Here's how the part is built. I have some questions about the finished solid (model axes, mm). A direction names the side the tool comes from. Round coordinates to 2 decimals unless told otherwise and drop trailing zeros. Loops run counter-clockwise (first coordinate to the right, second up) from the corner with the lowest first, then second, coordinate; pieces in that order, holes last. Notation, with made-up numbers: M 82.5,33 L 133.5,33 A33 cw 133.5,70 Z; hole C 8.25,14 d7. An arc over 180 degrees is marked long. Use a Markdown table: item, result.
```python
from build123d import *

# Parameters (mm, degrees)
F0_W            = 30
F0_H            = 40
F1_DEPTH        = 2
F2_W            = 14
F2_H            = 8
F3_DEPTH        = 10
F5_DEPTH        = 10
F6_R            = 5
F7_R            = 2.5
F8_W            = 15
F8_H            = 40
F8_W_2          = 9
F8_H_2          = 34
F9_DEPTH        = 2
F10_W           = 0.8
F10_H           = 34
F11_DEPTH       = 10
F12_W           = 9
F12_H           = 8
F13_DEPTH       = 2
F14_W           = 5
F14_H           = 2.75
F14_H_2         = 4
F15_DEPTH       = 10
F17_DEPTH       = 1
F18_W           = 9
F18_H           = 6
F19_DEPTH       = 2
F20_R           = 1
F22_D           = 5.5
F22_CBORE_D     = 6.5
F22_CBORE_DEPTH = 0


with BuildPart() as f1:
    # F0 (on Top) → F1 (new body)
    with BuildSketch(Plane.XY):
        Rectangle(F0_W, F0_H)
    extrude(amount=F1_DEPTH)

    # F2 (on face) → F3 (cut)
    with BuildSketch(Plane.XY.offset(2)):
        with Locations((0, 8)):
            Rectangle(F2_W, F2_H)
    extrude(amount=-F3_DEPTH, mode=Mode.SUBTRACT)

    # F4 (on face) → F5 (cut)
    with BuildSketch(Plane.XY.offset(2)):
        Polygon((-1, -4), (-7, -4), (-7, -20), (7, -20), align=None)
        Polygon((15, -4), (7, -4), (15, -20), align=None)
    extrude(amount=-F5_DEPTH, mode=Mode.SUBTRACT)

    # F6
    f6_edges = [f1.edges().sort_by_distance(p)[0] for p in [
        (15, -4, 1),
        (15, 20, 1),
        (-1, -4, 1),
    ]]
    fillet(f6_edges, radius=F6_R)

    # F7
    f7_edges = [f1.edges().sort_by_distance(p)[0] for p in [
        (7, 12, 1),
        (7, 4, 1),
    ]]
    fillet(f7_edges, radius=F7_R)

    # F8 (on face) → F9 (join)
    with BuildSketch(Plane.XY.offset(2)):
        with Locations((-22.5, 0)):
            Rectangle(F8_W, F8_H)
        with Locations((-22.5, 0)):
            Rectangle(F8_W_2, F8_H_2, mode=Mode.SUBTRACT)
    extrude(amount=-F9_DEPTH)

    # F10 (on face) → F11 (cut)
    with BuildSketch(Plane.XY.offset(2)):
        with Locations((-14.8, 0)):
            Rectangle(F10_W, F10_H)
    extrude(amount=-F11_DEPTH, mode=Mode.SUBTRACT)

    # F12 (on face) → F13 (join)
    with BuildSketch(Plane.XY.offset(2)):
        with Locations((-22.5, -12.75)):
            Rectangle(F12_W, F12_H)
        with Locations((-22.5, -4.25)):
            Rectangle(F12_W, F12_H)
        with Locations((-22.5, 4.25)):
            Rectangle(F12_W, F12_H)
        with Locations((-22.5, 12.75)):
            Rectangle(F12_W, F12_H)
    extrude(amount=-F13_DEPTH)

    # F14 (on face) → F15 (cut)
    with BuildSketch(Plane.XY.offset(2)):
        with Locations((-22.5, -15.375)):
            Rectangle(F14_W, F14_H)
        with Locations((-22.5, -10.125)):
            Rectangle(F14_W, F14_H)
        Polygon((-27, -2.25), (-27, -6.25), (-21, -2.25), align=None)
        Polygon((-23.9995513111, -6.25), (-18, -6.25), (-18, -2.25), align=None)
        Polygon((-21.5, 2.25), (-18, 2.25), (-18, 8.25), (-25, 8.25), (-25, 2.25), (-23.5, 2.25), (-23.5, 7.25), (-21.5, 7.25), align=None)
        with Locations((-22.5, 12.75)):
            Rectangle(F14_W, F14_H_2)
    extrude(amount=-F15_DEPTH, mode=Mode.SUBTRACT)

    # F16 (on face) → F17 (cut)
    with BuildSketch(Plane.XY.offset(2)):
        Polygon((-27.2, 17), (-27.2, -17), (-27, -17), (-27, -16.75), (-26.8, -16.75), (-26.8, -8.75), (-27, -8.75), (-27, -8.25), (-26.8, -8.25), (-26.8, -6.1166666667), (-27, -6.25), (-27, -2.25), (-26.8, -2.25), (-26.8, -0.25), (-27, -0.25), (-27, 0.25), (-26.8, 0.25), (-26.8, 8.25), (-27, 8.25), (-27, 8.75), (-26.8, 8.75), (-26.8, 16.75), (-27, 16.75), (-27, 17), align=None)
        Polygon((-18, -16.75), (-18, -17), (-17.8, -17), (-17.8, 17), (-18, 17), (-18, 16.75), (-18.2, 16.75), (-18.2, 8.75), (-18, 8.75), (-18, 2.25), (-18.2, 2.25), (-18.2, 0.25), (-18, 0.25), (-18, -0.25), (-18.2, -0.25), (-18.2, -2.3833433049), (-18, -2.25), (-18, -6.25), (-18.2, -6.25), (-18.2, -8.25), (-18, -8.25), (-18, -8.75), (-18.2, -8.75), (-18.2, -16.75), align=None)
    extrude(amount=-F17_DEPTH, mode=Mode.SUBTRACT)

    # F18 (on face) → F19 (join)
    with BuildSketch(Plane.XY.offset(2)):
        with Locations((-11, 23)):
            Rectangle(F18_W, F18_H)
    extrude(amount=-F19_DEPTH)

    # F20
    f20_edges = [f1.edges().sort_by_distance(p)[0] for p in [
        (-15.5, 26, 1),
        (-6.5, 26, 1),
        (-6.5, 20, 1),
        (-15.5, 20, 1),
    ]]
    fillet(f20_edges, radius=F20_R)

    # F22 (through all)
    with Locations(Plane.XY.offset(2)):
        with Locations((-11, 22)):
            CounterBoreHole(F22_D / 2, F22_CBORE_D / 2, F22_CBORE_DEPTH)


solid = f1.part
```
Q1. Will these pins go through, and if not, where does the flat tip stop? P1, Ø0.6, axis at x = -3.5, z = 1, coming from the -Y side; P2, Ø1, axis at x = -22.5, z = 1, coming from the +Y side.
Return value:
| item | result |
|---|---|
| P1 | stops at y = -4.08 |
| P2 | stops at y = 20 |
Q2. For faces 4 (the flat face through (-18.2, -1.3, 1.5)), 5 (the flat face through (-6, -4, 1)), 6 (the flat face through (-21, -6.25, 1)), 7 (the flat face through (11, -12, 1)), which set-ups out of +Z, -Z, +X, -X, +Y, -Y let a thin tool reach every point of the face, with its end or its side?
Return value:
| item | result |
|---|---|
| face 4 | +Z |
| face 5 | +Z, -Z, -Y |
| face 6 | +Z, -Z |
| face 7 | +Z, -Z, +X |
Q3. We'd pull the mould along Y, two halves only. Please class faces 1 (the flat face through (3.737, -13.475, 1.014)), 2 (the flat face through (-23, 3, 2)), 3 (the flat face through (-26.8, 4.2, 1.5)): pulls with the +Y half, pulls with the -Y half, needs draft (parallel to the pull), parting line crosses it, or undercut.
Return value:
| item | result |
|---|---|
| face 1 | pulls with the -Y half |
| face 2 | needs draft |
| face 3 | undercut |
Q4. I need wall thicknesses on line 1 (X direction, y = 8, z = 0.8); line 2 (X direction, y = 6.5, z = 0.45); line 3 (Y direction, x = -4.5, z = 0.1). Which ranges of each line are inside material? Lowest first, please. Write a range as from..to.
Return value:
| item | result |
|---|---|
| line 1 | x = -30..-25, -18..-15.2, -14.4..-7, 7..15 |
| line 2 | x = -30..-25, -23.5..-21.5, -18..-15.2, -14.4..-7, 7..15 |
| line 3 | y = -4..4, 12..20 |
Q5. Imagine slicing it at B-B, the plane z = 1.6. Give the number of separate pieces and of enclosed holes in the cut face, then the cut area to 3 significant figures.
Return value:
| item | result |
|---|---|
| separate pieces | 5 |
| enclosed holes | 5 |
| area | 1,320 mm^2 |
Q6. Imagine slicing it at A-A, the plane y = 22. Please give me the cut outline in (x, z), then the cut area to 3 significant figures.
Return value:
| item | result |
|---|---|
| outline | M -15.5,0 L -13.75,0 L -13.75,2 L -15.5,2 Z; M -8.25,0 L -6.5,0 L -6.5,2 L -8.25,2 Z |
| area | 7.00 mm^2 |
Q7. Imagine slicing it at C-C, the plane x = -11. Please give me the cut outline in (y, z), then the cut area to 3 significant figures.
Return value:
| item | result |
|---|---|
| outline | M -20,0 L 19.25,0 L 19.25,2 L -20,2 Z; M 24.75,0 L 26,0 L 26,2 L 24.75,2 Z |
| area | 81.0 mm^2 |
